Design review of the part shown in the three views and the two pictorial views. Dimensions are in mm from the part's minimum x, y and z. A direction names the side the tool comes from. Coordinates: 2 decimals unless noted, no trailing zeros. Loops run counter-clockwise (first coordinate to the right, second up) from the corner with the lowest first, then second, coordinate; pieces in that order, holes last. Notation, with made-up numbers: M 83.25,69 L 100.25,69 A20 cw 100.25,94 Z; hole C -26,-5 d2. An arc over 180 degrees is marked long. Use CSV: the item, a comma, the result in double quotes. Start each with the question number.
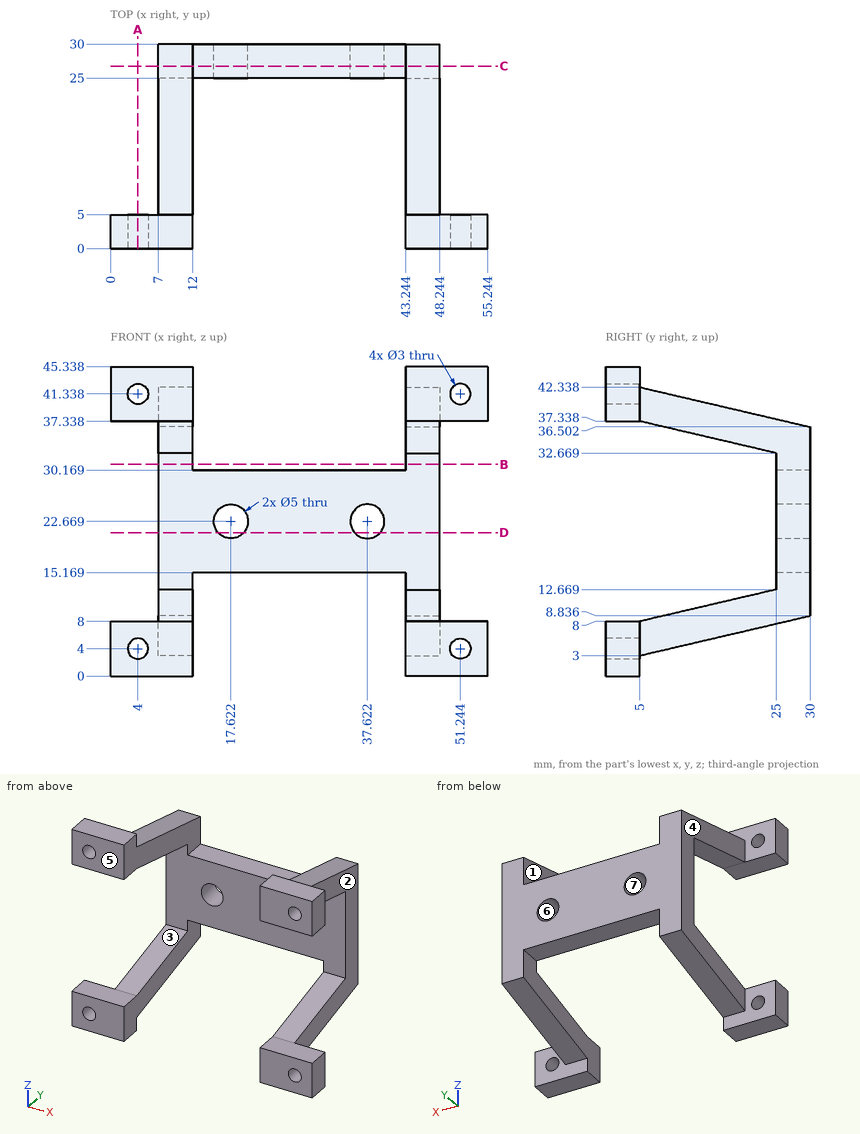
1. For the marked faces 1, 2 and 3, list the 3-axis set-ups (+Z, -Z, +X, -X, +Y, -Y) from which the entire face can be reached by the end or side of a thin tool; tool diameter is ignored.
2. To check wall thickness, follow line 1 along X through (y, z) = (1.5, 4); line 2 along X through (y, z) = (2, 6); line 3 along Z through (x, y) = (8.5, 3.5). State the ranges of each line that lie inside material, in increasing order.
3. Add section D-D (z = 21). Write out the cut boundary in (x, y), plus the area to 3 significant figures.
4. Insertion check: pin 1 Ø6 at (x, z) = (30.5, 21.5) entering from -Y; pin 2 Ø4 at (x, y) = (12.5, 14) entering from -Z; pin 3 Ø8 at (y, z) = (12, 35) entering from +X. Each pin has a flat end and moves straight along its axis. Give the tip position at first contact, or say it passes through.
5. Add section A-A (x = 4). Write out the cut boundary in (y, z), plus the area to 3 significant figures.
6. Add section C-C (y = 26.75). Write out the cut boundary in (x, z).
7. Add section B-B (z = 31). Write out the cut boundary in (x, y), plus the area to 3 significant figures.
8. Draft analysis for pull direction X (two halves, no side actions). For the marked faces 4, 5, 6 and 7, state which applies: released by +X, released by -X, zero draft, split by the parting line, or undercut.
Solved:
1,face 1,"+Z, +Y, -Y"
1,face 2,"+Z, -Z, +X, +Y"
1,face 3,"+X, -X, -Y"
2,line 1,"x = 0 to 2.5, 5.5 to 12, 43.24 to 49.74, 52.74 to 55.24"
2,line 2,"x = 0 to 12, 43.24 to 55.24"
2,line 3,"z = 0 to 8, 37.34 to 45.34"
3,outline,"M 7,25 L 15.76,25 L 15.76,30 L 7,30 Z; M 19.48,25 L 35.76,25 L 35.76,30 L 19.48,30 Z; M 39.48,25 L 48.24,25 L 48.24,30 L 39.48,30 Z"
3,area,"169 mm^2"
4,pin 1,"stops at y = 25"
4,pin 2,"stops at z = 4.65"
4,pin 3,"stops at x = 48.24"
5,outline,"M 0,0 L 5,0 L 5,2.5 L 0,2.5 Z; M 0,5.5 L 5,5.5 L 5,8 L 0,8 Z; M 0,37.34 L 5,37.34 L 5,39.84 L 0,39.84 Z; M 0,42.84 L 5,42.84 L 5,45.34 L 0,45.34 Z"
5,area,"50.0 mm^2"
6,outline,"M 7,8.08 L 12,8.08 L 12,15.17 L 43.24,15.17 L 43.24,8.08 L 48.24,8.08 L 48.24,37.26 L 43.24,37.26 L 43.24,30.17 L 12,30.17 L 12,37.26 L 7,37.26 Z; hole C 17.62,22.67 d5; hole C 37.62,22.67 d5"
7,outline,"M 7,25 L 12,25 L 12,30 L 7,30 Z; M 43.24,25 L 48.24,25 L 48.24,30 L 43.24,30 Z"
7,area,"50.0 mm^2"
8,face 4,"released by -X"
8,face 5,"zero draft"
8,face 6,"undercut"
8,face 7,"undercut"
